Model file for the job. Use its own axes, mm. Face numbers are marked on the shaded views. Give positions to 0.01 mm unless a question says otherwise; leave off trailing zeros. Order: outer loops, then holes, each group sorted by start corner. A loop starts at its lowest first (then second) coordinate and runs counter-clockwise, first axis right, second up. Notation, with made-up numbers: M -5,16.25 L 29,16.25 A27 ccw 29,36.25 Z; hole C 88.5,14.5 d7. An arc over 180 degrees is marked long. Return JSON: item names as keys, results as strings. Group by question number.
1. Slice it at C-C on z = -18.5. List the corners of the cut face in (x, y), then the cut area to 3 significant figures.
2. Two-plate mould, pull along Y, no slides. Class the marked faces 1, 2 and 3: released by +Y, released by -Y, zero draft, split by the parting line, or undercut.
3. Pin check, flat tips, straight feed: pin 1 (0.7 mm diameter, centred on x = 11.5, z = -24.5, fed in from +Y); pin 2 (2.5 mm diameter, centred on x = 12.5, y = 0, fed in from +Z); pin 3 (1.2 mm diameter, centred on x = -17, z = -24.5, fed in from -Y); pin 4 (5 mm diameter, centred on x = -30.5, y = -9, fed in from +Z). Stop position of each tip, or through.
4. Slice it at A-A on x = 12.5. List the corners of the cut face in (y, z), then the cut area to 3 significant figures.
5. Wall check: probe 1 along X at (y, z) = (0, -22.75); probe 2 along Y at (x, z) = (-12.5, -23.85); probe 3 along Y at (x, z) = (-32.5, -16.5). Give the ranges that are in metal, low to high. Write a range as [from, to].
6. Slice it at B-B on y = 0. List the corners of the cut face in (x, z).
7. Slice it at D-D on x = 22. List the corners of the cut face in (y, z).
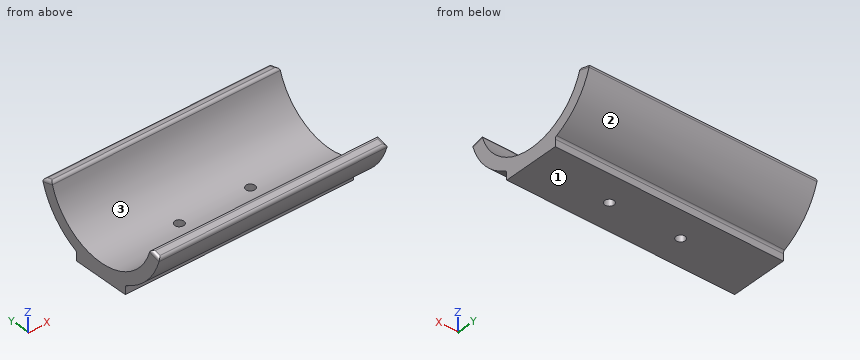
from build123d import *

# Parameters (mm, degrees)
BOSS_EXTRUDE1_DEPTH     = 40
CUT_EXTRUDE1_DEPTH      = 52.04942644
CUT_EXTRUDE1_DEPTH_BACK = 52.04942644
SKETCH2_R               = 1.6
FILLET1_R               = 1


with BuildPart() as part:
    # Sketch1 → Boss-Extrude1 (new, symmetric)
    with BuildSketch(Plane.YZ):
        with BuildLine():
            Line((20.284442352, -5.435199947), (24.148145657, -6.470476128))
            ThreePointArc((24.148145657, -6.470476128), (18.950253605, -16.306069064), (10, -22.912878475))
            Line((10, -22.912878475), (10, -26))
            Line((10, -26), (-10, -26))
            Line((-10, -26), (-10, -22.912878475))
            ThreePointArc((-10, -22.912878475), (-18.950253605, -16.306069064), (-24.148145657, -6.470476128))
            Line((-24.148145657, -6.470476128), (-20.284442352, -5.435199947))
            ThreePointArc((-20.284442352, -5.435199947), (0, -21), (20.284442352, -5.435199947))
        make_face()
    extrude(amount=BOSS_EXTRUDE1_DEPTH, both=True)

    # Sketch2 → Cut-Extrude1 (cut, two sides: drawn at the far end of the back side and taken through both)
    with BuildSketch(Plane(origin=(0, 0, -26), x_dir=(-1, 0, 0), z_dir=(0, 0, -1)).offset(-CUT_EXTRUDE1_DEPTH_BACK)):
        with Locations((12.5, 0)):
            Circle(SKETCH2_R)
        with Locations((-12.5, 0)):
            Circle(SKETCH2_R)
    extrude(amount=CUT_EXTRUDE1_DEPTH + CUT_EXTRUDE1_DEPTH_BACK, mode=Mode.SUBTRACT)

    # Fillet1
    fillet1_edges = [part.edges().sort_by_distance(p)[0] for p in [
        (-40, -22.216294005, -5.952838037),
        (0, 20.284442352, -5.435199947),
        (0, 24.148145657, -6.470476128),
        (0, 10, -22.912878475),
        (0, -10, -22.912878475),
        (0, -24.148145657, -6.470476128),
        (0, -20.284442352, -5.435199947),
        (40, 22.216294005, -5.952838037),
        (-40, 22.216294005, -5.952838037),
        (40, -22.216294005, -5.952838037),
    ]]
    fillet(fillet1_edges, radius=FILLET1_R)


solid = part.part
Result:
{
 "1": {"outline": "M -40,-16.82 L 40,-16.82 L 40,-9.94 L -40,-9.94 Z; M -40,9.94 L 40,9.94 L 40,16.82 L -40,16.82 Z", "area": "1,100 mm2"},
 "2": {"face 1": "zero draft", "face 2": "released by +Y", "face 3": "undercut"},
 "3": {"pin 1": "stops at y = 10", "pin 2": "passes through", "pin 3": "stops at y = -10", "pin 4": "stops at z = -17.57"},
 "4": {"outline": "M -23.86,-7.47 A25 ccw -10.58,-22.65 A1 cw -10,-23.56 L -10,-26 L -1.6,-26 L -1.6,-20.94 A21 cw -20.02,-6.35 A1 ccw -21.23,-5.69 L -23.16,-6.21 A1 ccw Z; M 1.6,-26 L 10,-26 L 10,-23.56 A1 cw 10.58,-22.65 A25 ccw 23.86,-7.47 A1 ccw 23.16,-6.21 L 21.23,-5.69 A1 ccw 20.02,-6.35 A21 cw 1.6,-20.94 Z", "area": "258 mm2"},
 "5": {"probe 1": "x = [-40, -14.1], [-10.9, 10.9], [14.1, 40]", "probe 2": "y = [-10, -1.6], [1.6, 10]", "probe 3": "y = [-18.78, -12.99], [12.99, 18.78]"},
 "6": {"outline": "M -40,-26 L -14.1,-26 L -14.1,-21 L -40,-21 Z; M -10.9,-26 L 10.9,-26 L 10.9,-21 L -10.9,-21 Z; M 14.1,-26 L 40,-26 L 40,-21 L 14.1,-21 Z"},
 "7": {"outline": "M -23.86,-7.47 A25 ccw -10.58,-22.65 A1 cw -10,-23.56 L -10,-26 L 10,-26 L 10,-23.56 A1 cw 10.58,-22.65 A25 ccw 23.86,-7.47 A1 ccw 23.16,-6.21 L 21.23,-5.69 A1 ccw 20.02,-6.35 A21 cw -20.02,-6.35 A1 ccw -21.23,-5.69 L -23.16,-6.21 A1 ccw Z"}
}
